Geometry: final body of the model. Coordinates: model frame, mm. Face numbers are marked on the shaded views. Coordinates: 2 decimals unless noted, no trailing zeros. Loops run counter-clockwise (first coordinate to the right, second up) from the corner with the lowest first, then second, coordinate; pieces in that order, holes last. Notation, with made-up numbers: (70, 51) -> (79, 51) arc R21 ccw to (79, 90) -> close; hole circle Ø10 at (-19.75, 11.5). An arc over 180 degrees is marked (long way). One line per item, written item: value. Start each with the question number.
Item 1: Ray query, probe 1 along Y at (x, z) = (107.5, -64); probe 2 along Z at (x, y) = (0, 26). Return the intervals inside material, ascending. Write a range as from..to.
Item 2: Contact query for flat-ended pins moving along their axis: pin 1 Ø4 at (y, z) = (22, -47.5) entering from +X; pin 2 Ø10 at (y, z) = (-43, -133.5) entering from +X; pin 3 Ø10 at (x, y) = (99, -158.5) entering from -Z. Output: stop coordinate, or through.
Item 3: Mould query, pull axis X, two halves, no side actions, for the marked faces 1, 2 and 3. Classes: +X half, -X half, draft (parallel to the pull), parting line (faces both ways), or undercut.
Item 4: Section query C-C on y = 22. Return loops of the section in (x, z), then the cut area to 3 significant figures.
Item 5: Section query B-B on z = 137.5. Return loops of the section in (x, y).
Item 6: Section query A-A on x = 0. Return loops of the section in (y, z).
Item 7: Section query D-D on x = -124.5. Return loops of the section in (y, z).
from build123d import *

# Parameters (mm, degrees)
SKETCH1_R           = 100
BOSS_EXTRUDE1_DEPTH = 98
SKETCH3_R           = 98
CUT_EXTRUDE2_DEPTH  = 397
SKETCH5_R           = 175
SKETCH5_R_2         = 98
BOSS_EXTRUDE2_DEPTH = 2
SKETCH7_R           = 175
SKETCH7_R_2         = 173
BOSS_EXTRUDE3_DEPTH = 300
SKETCH8_R           = 175
BOSS_EXTRUDE4_DEPTH = 2


with BuildPart() as part:
    # Sketch1 → Boss-Extrude1 (new body)
    with BuildSketch(Plane(origin=(0, 0, 0), x_dir=(1, 0, 0), z_dir=(0, 1, 0))):
        Circle(SKETCH1_R)
    extrude(amount=BOSS_EXTRUDE1_DEPTH)

    # Sketch3 → Cut-Extrude2 (cut)
    with BuildSketch(Plane(origin=(0, 98, 0), x_dir=(1, 0, 0), z_dir=(0, 1, 0))):
        Circle(SKETCH3_R)
    extrude(amount=-CUT_EXTRUDE2_DEPTH, mode=Mode.SUBTRACT)

    # Sketch5 → Boss-Extrude2 (add)
    with BuildSketch(Plane.XZ):
        Circle(SKETCH5_R)
        Circle(SKETCH5_R_2, mode=Mode.SUBTRACT)
    extrude(amount=BOSS_EXTRUDE2_DEPTH)

    # Sketch7 → Boss-Extrude3 (add)
    with BuildSketch(Plane.XZ.offset(2)):
        Circle(SKETCH7_R)
        Circle(SKETCH7_R_2, mode=Mode.SUBTRACT)
    extrude(amount=BOSS_EXTRUDE3_DEPTH)

    # Sketch8 → Boss-Extrude4 (add)
    with BuildSketch(Plane.XZ.offset(302)):
        Circle(SKETCH8_R)
    extrude(amount=-BOSS_EXTRUDE4_DEPTH)


solid = part.part
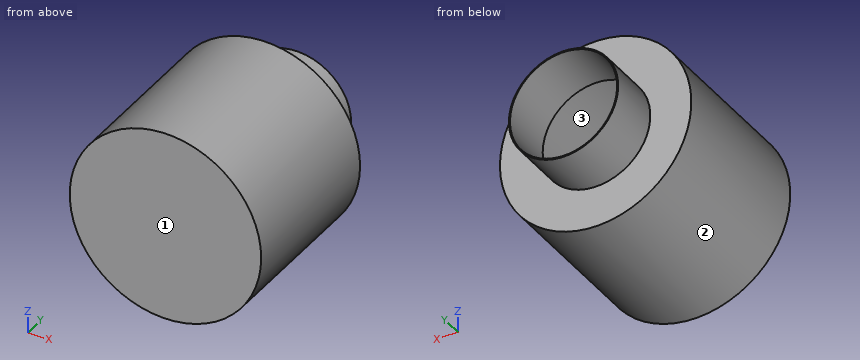
Reply:
1. probe 1: y = -302..-300, -2..0
1. probe 2: z = -100..-98, 98..100
2. pin 1: stops at x = 89.05
2. pin 2: stops at x = 118.8
2. pin 3: stops at z = -147.61
3. face 1: draft
3. face 2: parting line
3. face 3: undercut
4. outline: circle Ø200 at (0, 0); hole circle Ø196 at (0, 0)
4. area: 1,240 mm²
5. outline: (-108.25, -302) -> (108.25, -302) -> (108.25, 0) -> (-108.25, 0) -> close; hole (-104.99, -300) -> (104.99, -300) -> (104.99, -2) -> (-104.99, -2) -> close
6. outline: (-302, -175) -> (0, -175) -> (0, -100) -> (98, -100) -> (98, -98) -> (-2, -98) -> (-2, -173) -> (-300, -173) -> (-300, 173) -> (-2, 173) -> (-2, 98) -> (98, 98) -> (98, 100) -> (0, 100) -> (0, 175) -> (-302, 175) -> close
7. outline: (-302, -122.98) -> (0, -122.98) -> (0, 122.98) -> (-302, 122.98) -> close; hole (-300, -120.12) -> (-2, -120.12) -> (-2, 120.12) -> (-300, 120.12) -> close
